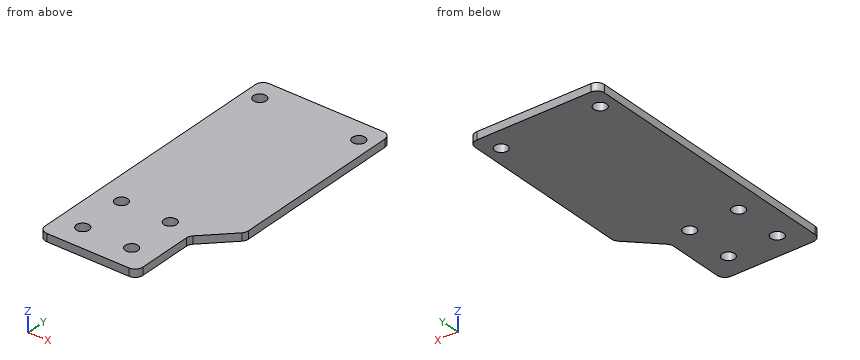
Autodesk Inventor part; units mm, degrees
ref_plane "YZ Plane" through (0, 0, 0) normal (1, 0, 0) x (0, 1, 0)
ref_plane "XZ Plane" through (0, 0, 0) normal (0, 1, 0) x (-1, 0, 0)
ref_plane "XY Plane" through (0, 0, 0) normal (0, 0, 1) x (1, 0, 0)
sketch "Sketch1" plane through (0, 0, 0) normal (0, 0, 1) x (1, 0, 0)
  line L0 (0, 0) -> (-40, 0)
  line L1 (-40, 0) -> (-40, 40)
  line L2 (-40, 40) -> (0, 40)
  line L3 (0, 40) -> (0, 0)
  line L4 (-30, 30) -> (-10, 30) construction
  line L5 (-10, 30) -> (-10, 10) construction
  line L6 (-10, 10) -> (-30, 10) construction
  line L7 (-30, 10) -> (-30, 30) construction
  line L8 (-30, 30) -> (-40, 30) construction
  line L9 (-10, 10) -> (0, 10) construction
  circle A0 centre (-30, 30) radius 2.6
  circle A1 centre (-10, 30) radius 2.6
  circle A2 centre (-10, 10) radius 2.6
  circle A3 centre (-30, 10) radius 2.6
  line L10 (-40, 40) -> (13, 40)
  line L11 (13, 40) -> (13, 102.4)
  line L12 (13, 102.4) -> (-40, 102.4)
  line L13 (-40, 102.4) -> (-40, 40)
  line L14 (13, 40) -> (0, 27)
  line L15 (-40, 102.4) -> (13, 102.4)
  line L16 (13, 102.4) -> (13, 122.4)
  line L17 (-40, 122.4) -> (-40, 102.4)
  line L18 (6.75, 122.4) -> (6.75, 115.12)
  line L19 (6.75, 115.12) -> (-33.75, 115.12)
  line L20 (-33.75, 115.12) -> (-33.75, 122.4)
  line L21 (-33.75, 115.12) -> (-40, 115.12)
  line L22 (6.75, 115.12) -> (13, 115.12)
  line L23 (-40, 122.4) -> (-33.75, 122.4)
  line L24 (13, 122.4) -> (6.75, 122.4)
  line L25 (-13.5, 115.12) -> (-13.5, 113.62) construction
  arc A4 (-18.2697, 115.12) -> (-8.7303, 115.12) centre (-13.5, 113.62) ccw
  dimension "d0" = 40
  dimension "d1" = 40
  dimension "d2" = 5.2
  dimension "d3" = 5.2
  dimension "d4" = 5.2
  dimension "d5" = 5.2
  dimension "d6" = 20
  dimension "d7" = 20
  dimension "d8" = 10
  dimension "d9" = 62.4
  dimension "d10" = 53
  dimension "d11" = 45
  dimension "d12" = 20
  dimension "d13" = 40.5
  dimension "d14" = 7.28
  dimension "d15" = 1.5
  dimension "d16" = 10
  dimension "d17" = 20
extrude "Extrusion1" add sketch "Sketch1" along normal blind 3.175 contours L0 L1 L2 L3 | L3 L10 L14 | L13 L12 L11 L10 L2 | L17 L21 L19 A4 L22 L16 L12 | L19 A4
fillet "Fillet1" radius 3.175 6 edges at (0, 0, 1.5875) (-40, 0, 1.5875) (0, 27, 1.5875) (13, 40, 1.5875) (-40, 115.12, 1.5875) (13, 115.12, 1.5875)
sketch "Sketch2" plane through (0, 0, 3.175) normal (0, 0, 1) x (1, 0, 0)
  line L0 (13, 41.3151) -> (13, 111.945) construction
  line L1 (-40, 118.604) -> (13, 118.604) construction
  line L2 (13, 118.604) -> (13, 98.604) construction
  line L3 (13, 98.604) -> (-40, 98.604) construction
  line L4 (-40, 98.604) -> (-40, 118.604) construction
  circle A0 centre (-33.75, 106.36) radius 2.6
  circle A1 centre (6.75, 106.36) radius 2.6
  line L5 (9.825, 115.12) -> (-36.825, 115.12) construction
  line L6 (-33.75, 106.36) -> (-33.75, 115.12) construction
  line L7 (9.825, 115.12) -> (-36.825, 115.12) construction
  line L8 (6.75, 106.36) -> (6.75, 115.12) construction
  point P0 (0, 0)
  point P1 (13, 121.9)
  point P2 (-18.2697, 115.12)
  point P3 (-8.7303, 115.12)
  point P4 (13, 115.12)
  point P5 (-40, 115.12)
  dimension "d22" = 20
  dimension "d23" = 5.2
  dimension "d24" = 5.2
  dimension "d25" = 8.76
  dimension "d26" = 8.76
  dimension "d29" = 3.484
extrude "Extrusion2" cut sketch "Sketch2" against normal up to next
equation "\"d3\" = d2"
equation "\"d4\" = d2"
equation "\"d5\" = d2"
equation "\"d24\" = d23"
equation "\"d26\" = d25"
properties part number "X Axis Statonary NON ADJUSTABLE Composite Belt Holder"
Geometry check sheet. Reference: the model listing, model coordinates, mm. Give positions to 0.01 mm unless a question says otherwise; leave off trailing zeros. Order: outer loops, then holes, each group sorted by start corner. A loop starts at its lowest first (then second) coordinate and runs counter-clockwise, first axis right, second up. Notation, with made-up numbers: (-11.5, -2.75) - (35.5, -2.75) arc R20 ccw to (35.5, 5.25) - close; hole circle Ø4 at (-25.5, -9.75). An arc over 180 degrees is marked (long way). Answer in a Markdown table with one row per item. Add a question column.
Q1. Cross-section at A-A, the plane y = 106.36. Enter the section's corners in (x, z) (3 decimals), then the cut area to 3 significant figures.
Q2. Cross-section at D-D, the plane z = 1.6. Enter the section's corners in (x, y) (3 decimals), then the cut area to 3 significant figures.
Q3. Material ranges on probe 1 along Y at (x, z) = (-10, 1.85); probe 2 along Y at (x, z) = (-8, 1.45); probe 3 along Y at (x, z) = (-33.75, 1.8), recorded low to high. Write a range as from..to.
Q4. Gauge pin test, flat end, axial feed: pin 1 (1 mm diameter, centred on y = 13.5, z = 1, fed in from +X). Record the tip position at first contact, or that the pin passes through.
Q5. Cross-section at C-C, the plane x = -11. Enter the section's corners in (y, z) (3 decimals).
Q6. Cross-section at B-B, the plane x = 6.75. Enter the section's corners in (y, z) (3 decimals).
Check values:
| question | item | result |
|---|---|---|
| 1 | outline | (-40, 0) - (-36.35, 0) - (-36.35, 3.175) - (-40, 3.175) - close; (-31.15, 0) - (4.15, 0) - (4.15, 3.175) - (-31.15, 3.175) - close; (9.35, 0) - (13, 0) - (13, 3.175) - (9.35, 3.175) - close |
| 1 | area | 135 mm^2 |
| 2 | outline | (-40, 3.175) arc R3.175 ccw to (-36.825, 0) - (-3.175, 0) arc R3.175 ccw to (0, 3.175) - (0, 25.685) arc R3.175 cw to (0.93, 27.93) - (12.07, 39.07) arc R3.175 ccw to (13, 41.315) - (13, 111.945) arc R3.175 ccw to (9.825, 115.12) - (-36.825, 115.12) arc R3.175 ccw to (-40, 111.945) - close; hole circle Ø5.2 at (-33.75, 106.36); hole circle Ø5.2 at (-30, 10); hole circle Ø5.2 at (-30, 30); hole circle Ø5.2 at (-10, 10); hole circle Ø5.2 at (-10, 30); hole circle Ø5.2 at (6.75, 106.36) |
| 2 | area | 5,530 mm^2 |
| 3 | probe 1 | y = 0..7.4, 12.6..27.4, 32.6..115.12 |
| 3 | probe 2 | y = 0..8.34, 11.66..28.34, 31.66..115.12 |
| 3 | probe 3 | y = 0..103.76, 108.96..115.12 |
| 4 | pin 1 | stops at x = 0 |
| 5 | outline | (0, 0) - (7.6, 0) - (7.6, 3.175) - (0, 3.175) - close; (12.4, 0) - (27.6, 0) - (27.6, 3.175) - (12.4, 3.175) - close; (32.4, 0) - (115.12, 0) - (115.12, 3.175) - (32.4, 3.175) - close |
| 6 | outline | (33.75, 0) - (103.76, 0) - (103.76, 3.175) - (33.75, 3.175) - close; (108.96, 0) - (115.12, 0) - (115.12, 3.175) - (108.96, 3.175) - close |
